```python
from build123d import *

# Parameters (mm, degrees)
F1_W        = 45
F1_H        = 35
F1_W_2      = 12
F1_H_2      = 24
F2_DEPTH    = 2
F3_T1_DEPTH = 55
F4_T1_DEPTH = 55
F5_T1_DEPTH = 37
F5_T4_ANGLE = 196.3896000127
F5_T6_ANGLE = 196.3896000127
F6_T1_DEPTH = 37
F6_T4_ANGLE = 196.3896000127
F6_T6_ANGLE = 196.3896000127


# Not quite as in the source:
# - a fillet or chamfer that OpenCascade refuses, or shapes differently, is made with other operations: its cross-section is extruded or revolved along the edge and cut away or added


with BuildPart() as f2:
    # F1 (on face) → F2 (new body)
    with BuildSketch(Plane.XY):
        with Locations((-7.2387225181, -9.9369412684)):
            Rectangle(F1_W, F1_H)
        with Locations((-18.7387225181, -9.9369412684)):
            Rectangle(F1_W_2, F1_H_2, mode=Mode.SUBTRACT)
        with Locations((4.2612774819, -9.9369412684)):
            Rectangle(F1_W_2, F1_H_2, mode=Mode.SUBTRACT)
    extrude(amount=F2_DEPTH)

    # F3: fillet of radius 5 on 1 edges, made by hand

    # F3_s2 → F3_t1 (cut)
    with BuildSketch(Plane.XZ.offset(-17.5630587316)):
        with BuildLine():
            ThreePointArc((-29.7387225181, 0), (-27.9747904956, 1.472135955), (-25.7387225181, 2))
            Line((-25.7387225181, 2), (-29.7387225181, 2))
            Line((-29.7387225181, 2), (-29.7387225181, 0))
        make_face()
    extrude(amount=F3_T1_DEPTH, mode=Mode.SUBTRACT)

    # F4: fillet of radius 5 on 1 edges, made by hand

    # F4_s2 → F4_t1 (cut)
    with BuildSketch(Plane.XZ.offset(-17.5630587316)):
        with BuildLine():
            ThreePointArc((15.2612774819, 0), (13.4973454594, 1.472135955), (11.2612774819, 2))
            Line((11.2612774819, 2), (15.2612774819, 2))
            Line((15.2612774819, 2), (15.2612774819, 0))
        make_face()
    extrude(amount=F4_T1_DEPTH, mode=Mode.SUBTRACT)

    # F5: fillet of radius 5 on 1 edges, made by hand

    # F5_s2 → F5_t1 (cut)
    with BuildSketch(Plane.YZ.offset(-25.7387225181)):
        with BuildLine():
            ThreePointArc((-27.4369412684, -3), (-25.9724751743, 0.5355339059), (-22.4369412684, 2))
            Line((-22.4369412684, 2), (-27.4369412684, 2))
            Line((-27.4369412684, 2), (-27.4369412684, -3))
        make_face()
    extrude(amount=F5_T1_DEPTH, mode=Mode.SUBTRACT)

    # F5_s3 → F5_t4 (revolve, cut)
    with BuildSketch(Plane(origin=(-24.5015511946, 0, -7.2063663149), x_dir=(0, 1, 0), z_dir=(0.9593652077, 0, 0.2821673233))):
        with BuildLine():
            ThreePointArc((-22.4369412684, -0.615469186), (-25.9724751743, 0.848996908), (-27.4369412684, 4.384530814))
            Line((-27.4369412684, 4.384530814), (-27.4369412684, -0.615469186))
            Line((-27.4369412684, -0.615469186), (-22.4369412684, -0.615469186))
        make_face()
    revolve(axis=Axis((-25.7387225181, -27.4369412684, -3), (0, 1, 0)), revolution_arc=F5_T4_ANGLE, mode=Mode.SUBTRACT)

    # F5_s5 → F5_t6 (revolve, cut)
    with BuildSketch(Plane.YZ.offset(11.2612774819)):
        with BuildLine():
            ThreePointArc((-22.4369412684, 2), (-25.9724751743, 0.5355339059), (-27.4369412684, -3))
            Line((-27.4369412684, -3), (-27.4369412684, 2))
            Line((-27.4369412684, 2), (-22.4369412684, 2))
        make_face()
    revolve(axis=Axis((11.2612774819, -27.4369412684, -3), (0, 1, 0)), revolution_arc=F5_T6_ANGLE, mode=Mode.SUBTRACT)

    # F6: fillet of radius 5 on 1 edges, made by hand

    # F6_s2 → F6_t1 (cut)
    with BuildSketch(Plane.YZ.offset(-25.7387225181)):
        with BuildLine():
            ThreePointArc((7.5630587316, -3), (6.0985926376, 0.5355339059), (2.5630587316, 2))
            Line((2.5630587316, 2), (7.5630587316, 2))
            Line((7.5630587316, 2), (7.5630587316, -3))
        make_face()
    extrude(amount=F6_T1_DEPTH, mode=Mode.SUBTRACT)

    # F6_s3 → F6_t4 (revolve, cut)
    with BuildSketch(Plane.YZ.offset(11.2612774819)):
        with BuildLine():
            ThreePointArc((7.5630587316, -3), (6.0985926376, 0.5355339059), (2.5630587316, 2))
            Line((2.5630587316, 2), (7.5630587316, 2))
            Line((7.5630587316, 2), (7.5630587316, -3))
        make_face()
    revolve(axis=Axis((11.2612774819, 7.5630587316, -3), (0, 1, 0)), revolution_arc=F6_T4_ANGLE, mode=Mode.SUBTRACT)

    # F6_s5 → F6_t6 (revolve, cut)
    with BuildSketch(Plane(origin=(-24.5015511946, 0, -7.2063663149), x_dir=(0, 1, 0), z_dir=(0.9593652077, 0, 0.2821673233))):
        with BuildLine():
            ThreePointArc((2.5630587316, -0.615469186), (6.0985926376, 0.848996908), (7.5630587316, 4.384530814))
            Line((7.5630587316, 4.384530814), (7.5630587316, -0.615469186))
            Line((7.5630587316, -0.615469186), (2.5630587316, -0.615469186))
        make_face()
    revolve(axis=Axis((-25.7387225181, 7.5630587316, -3), (0, 1, 0)), revolution_arc=F6_T6_ANGLE, mode=Mode.SUBTRACT)


solid = f2.part
```
Work out the finished part from the listing and answer in its coordinate system (mm). A direction names the side the tool comes from. Give positions to 0.01 mm unless a question says otherwise; leave off trailing zeros. Loops run counter-clockwise (first coordinate to the right, second up) from the corner with the lowest first, then second, coordinate; pieces in that order, holes last. Notation, with made-up numbers: (52.5, 21) - (97.5, 21) arc R19 cw to (97.5, 34) - close; hole circle Ø10 at (-38.5, -36). An arc over 180 degrees is marked (long way). One line per question, with ' | ' between items.
(1) The part is cut by section A-A (x = -1). Write down the section's boundary in (y, z).
Recorded:
outline: (-26.44, 0) - (-21.94, 0) - (-21.94, 2) - (-22.44, 2) arc R5 ccw to start; (2.06, 0) - (6.56, 0) arc R5 ccw to (2.56, 2) - (2.06, 2) - close
(2) Each of these flat-tipped pins is pushed along its axis until it touches: pin 1 Ø1 at (y, z) = (-15.5, 1) entering from +X; pin 2 Ø1 at (x, z) = (-20.5, 1.5) entering from +Y; pin 3 Ø1 at (x, z) = (5, 1) entering from +Y. Where does it stop, or does it pass through?
Recorded:
pin 1: stops at x = 14.83 | pin 2: stops at y = 5.56 | pin 3: stops at y = 6.13
(3) The mould has two halves that part along X. Classify faces 3 (the face through (-7.498, 4.828, 1.458)), 4 (the face through (-28, -9.76, 1.46)), 5 (the face through (13.526, -9.762, 1.458)), 6 (the face through (-12.739, -10, 1)): +X half, -X half, draft (parallel to the pull), parting line (faces both ways), or undercut.
Recorded:
face 3: draft | face 4: -X half | face 5: +X half | face 6: undercut
(4) The part is cut by section B-B (y = -12). Write down the section's boundary in (x, z).
Recorded:
outline: (-29.74, 0) - (-24.74, 0) - (-24.74, 2) - (-25.74, 2) arc R5 ccw to start; (-12.74, 0) - (-1.74, 0) - (-1.74, 2) - (-12.74, 2) - close; (10.26, 0) - (15.26, 0) arc R5 ccw to (11.26, 2) - (10.26, 2) - close
(5) The part is cut by section D-D (x = -10). Write down the section's boundary in (y, z).
Recorded:
outline: (-26.44, 0) - (6.56, 0) arc R5 ccw to (2.56, 2) - (-22.44, 2) arc R5 ccw to start
(6) Straight lines are drawn through the part: probe 1 along X at (y, z) = (-1.5, 1.25); probe 2 along X at (y, z) = (2, 1.5); probe 3 along Z at (x, y) = (-26, 2.5). For each, find the intervals that lie inside material, in ascending order.
Recorded:
probe 1: x = -28.37 to -24.74, -12.74 to -1.74, 10.26 to 13.9 | probe 2: x = -27.92 to -24.74, -12.74 to -1.74, 10.26 to 13.44 | probe 3: z = 0 to 1.99
(7) The part is cut by section C-C (z = 0.9). Write down the section's boundary in (x, y), then the cut area to 3 significant figures.
Recorded:
outline: (-28.87, -22.44) arc R3.13 ccw to (-25.74, -25.57) - (11.26, -25.57) arc R3.13 ccw to (14.39, -22.44) - (14.39, 2.56) arc R3.13 ccw to (11.26, 5.69) - (-25.74, 5.69) arc R3.13 ccw to (-28.87, 2.56) - close; hole (-24.74, -21.94) - (-12.74, -21.94) - (-12.74, 2.06) - (-24.74, 2.06) - close; hole (-1.74, -21.94) - (10.26, -21.94) - (10.26, 2.06) - (-1.74, 2.06) - close | area: 768 mm²
(8) A tool of negligible diameter and unlimited length cuts with its end or side. For faces 1 (the face through (-7.5, -24.7, 1.46)), 2 (the face through (10.261, -10, 1)), from which of +Z, -Z, +X, -X, +Y, -Y can it reach the whole face along a straight path? Write none if from no direction.
Recorded:
face 1: +Z, +X, -X, -Y | face 2: +Z, -Z
